Autodesk Inventor part; units mm, degrees
ref_plane "YZ Plane" through (0, 0, 0) normal (1, 0, 0) x (0, 1, 0)
ref_plane "XZ Plane" through (0, 0, 0) normal (0, 1, 0) x (-1, 0, 0)
ref_plane "XY Plane" through (0, 0, 0) normal (0, 0, 1) x (1, 0, 0)
sketch "Szkic1" plane through (0, 0, 0) normal (0, 0, 1) x (1, 0, 0)
  line L0 (-21, 0) -> (21, 0) construction
  line L1 (0, -28) -> (0, 28) construction
  circle A0 centre (0, 0) radius 3
  circle A1 centre (0, 0) radius 5.05
  line L2 (15, 20) -> (-15, 20)
  line L3 (-15, 20) -> (-15, -20)
  line L4 (-15, -20) -> (15, -20)
  line L5 (15, -20) -> (15, 20)
  line L6 (15, 20) -> (-15, -20) construction
  line L7 (-15, 20) -> (15, -20) construction
  line L8 (5.05, 2.9156) -> (5.05, -2.9156)
  line L9 (0, 5.8312) -> (5.05, 2.9156)
  line L10 (-5.05, 2.9156) -> (0, 5.8312)
  line L11 (-5.05, -2.9156) -> (-5.05, 2.9156)
  line L12 (0, -5.8312) -> (-5.05, -2.9156)
  line L13 (5.05, -2.9156) -> (0, -5.8312)
  point P0 (5.05, -2.9156)
  dimension "d0" = 6
  dimension "d1" = 10.1
  dimension "d2" = 30
  dimension "d3" = 40
  dimension "d8" = 360
extrude "Wyciągnięcie proste1" add sketch "Szkic1" along normal blind 20 contours A1 | L8 L13 A1 | A1 L9 L8 | A1 L10 L9 | L13 L12 A1 | A1 L11 L10 | L12 L11 A1 | L5 L4 L3 L2
extrude "Wyciągnięcie proste2" add sketch "Szkic1" against normal blind 5 contours L5 L4 L3 L2
fillet "Zaokrąglenie1" radius 1 6 edges at (5.05, 0, -5) (2.525, 4.3734, -5) (-2.525, 4.3734, -5) (-5.05, 0, -5) (-2.525, -4.3734, -5) (2.525, -4.3734, -5)
sketch "Szkic2" plane through (-15, -20, 20) normal (-1, 0, 0) x (0, 0, 1)
  line L0 (-25, 0) -> (-25, 40)
  line L1 (-20, -8) -> (-20, 48) construction
  line L2 (-30.5, 20) -> (8, 20) construction
  circle A0 centre (-12.5, 31) radius 3
  circle A1 centre (-12.5, 9) radius 3
  circle A2 centre (-12.5, 31) radius 7.5
  circle A3 centre (-12.5, 9) radius 7.5
  point P0 (-20, 20)
  dimension "d14" = 6
  dimension "d15" = 7.5
  dimension "d16" = 11
  dimension "d17" = 15
extrude "Wyciągnięcie proste3" cut sketch "Szkic2" against normal through all contours A0 | A1
hole "Otwór1" at (-15, -11, 7.5) at (-15, 11, 7.5) direction (1, 0, 0) diameter 6.2 end through all
hole "Otwór2" at (0, 0, 0) direction (0, 0, -1) diameter 6.2 end through all
hole "Otwór3" at (0, 0, 0) direction (0, 0, 1) diameter 6.2 end through all
properties part number "uMule-Uchwyt_koła"
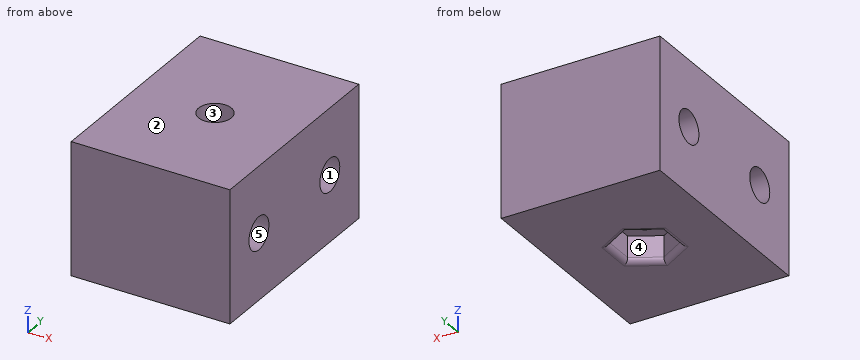
Design review of the part built by this model. Coordinates are the model's own, in mm. Face numbers are marked on the shaded views. A direction names the side the tool comes from. Give positions to 0.01 mm unless a question says otherwise; leave off trailing zeros. Order: outer loops, then holes, each group sorted by start corner. A loop starts at its lowest first (then second) coordinate and runs counter-clockwise, first axis right, second up. Notation, with made-up numbers: (89, 65) - (111, 65) arc R24 ccw to (111, 92) - close; hole circle Ø7 at (64, 84.5). An arc over 180 degrees is marked (long way). Use a Markdown table: item, result. Add a question column.
(1) Add section C-C on x = 7.5. Give the boundary of the cut face in (y, z), then the cut area to 3 significant figures.
(2) Wall thickness on probe 1 along Y at (x, z) = (0, 7.25); probe 2 along Y at (x, z) = (-6.5, 6); probe 3 along Y at (x, z) = (0, 11): over which ranges is each line inside the solid? List them lowest first. Write a range as [from, to].
(3) Add section A-A on z = 7.5. Give the boundary of the cut face in (x, y).
(4) Mouldability with a two-part tool opening along Z and no side actions: class the marked faces 1, 2 and 3 as +Z half, -Z half, draft (parallel to the pull), parting line (faces both ways), or undercut.
(5) Clearance check with flat-ended pins moving along their axes: P1, Ø3.5, axis at y = 11, z = 7.5, coming from the +X side; P2, Ø11, axis at x = -2.5, y = 1, coming from the -Z side. State where each tip first meets the part, or that it passes through.
(6) Add section B-B on y = -11. Give the boundary of the cut face in (x, z), then the cut area to 3 significant figures.
(7) Machinability: for the marked faces 4 and 5, which of the approach directions +Z, -Z, +X, -X, +Y, -Y give a long, thin tool a straight path to every point of the face, cutting with its end or side? Answer none if there is none.
(8) Add section D-D on z = 12. Give the boundary of the cut face in (x, y).
Report:
| question | item | result |
|---|---|---|
| 1 | outline | (-20, -5) - (20, -5) - (20, 20) - (-20, 20) - close; hole circle Ø6.2 at (-11, 7.5); hole circle Ø6.2 at (11, 7.5) |
| 1 | area | 940 mm² |
| 2 | probe 1 | y = [-20, -14.09], [-7.91, -3.1], [3.1, 7.91], [14.09, 20] |
| 2 | probe 2 | y = [-20, -13.71], [-8.29, 8.29], [13.71, 20] |
| 2 | probe 3 | y = [-20, -3.1], [3.1, 20] |
| 3 | outline | (-15, -20) - (15, -20) - (15, -14.1) - (-15, -14.1) - close; (-15, -7.9) - (15, -7.9) - (15, 7.9) - (-15, 7.9) - close; (-15, 14.1) - (15, 14.1) - (15, 20) - (-15, 20) - close; hole circle Ø6.2 at (0, 0) |
| 4 | face 1 | undercut |
| 4 | face 2 | +Z half |
| 4 | face 3 | draft |
| 5 | P1 | passes through |
| 5 | P2 | stops at z = -5 |
| 6 | outline | (-15, -5) - (15, -5) - (15, 4.4) - (-15, 4.4) - close; (-15, 10.6) - (15, 10.6) - (15, 20) - (-15, 20) - close |
| 6 | area | 564 mm² |
| 7 | face 4 | -Z |
| 7 | face 5 | +X, -X |
| 8 | outline | (-15, -20) - (15, -20) - (15, 20) - (-15, 20) - close; hole circle Ø6.2 at (0, 0) |
